Read the model definition and answer for the solid it produces. Units are mm, in the model's axes. Give positions to 0.01 mm unless a question says otherwise; leave off trailing zeros. Loops run counter-clockwise (first coordinate to the right, second up) from the corner with the lowest first, then second, coordinate; pieces in that order, holes last.
(1) Find section B-B, the plane x = 0. Write down the section's boundary in (y, z) (3 decimals).
(2) Each of these flat-tipped pins is pushed along its axis until it touches: P1, Ø5, axis at y = 3, z = 165.5, coming from the +X side; P2, Ø6, axis at y = 4, z = 248.5, coming from the +X side (3 decimals). Where does it stop, or does it pass through?
(3) Find section A-A, the plane z = 233. Write down the section's boundary in (x, y) (3 decimals).
(4) Straight lines are drawn through the part: probe 1 along Y at (x, z) = (0, 249) (3 decimals); probe 2 along Y at (x, z) = (-1, 422); probe 3 along X at (y, z) = (-2.25, 384.5). For each, find the intervals that lie inside material, in ascending order.
```python
from build123d import *

# Parameters (mm, degrees)
BOSS_EXTRUDE1_DEPTH     = 514.48335
SKETCH2_R               = 3.175
CUT_EXTRUDE1_DEPTH      = 1
CUT_EXTRUDE1_DEPTH_BACK = 515.48335


with BuildPart() as part:
    # Sketch1 → Boss-Extrude1 (new body)
    with BuildSketch(Plane.XY):
        Polygon((-7.332348419, 0), (-3.666174209, -6.35), (3.666174209, -6.35), (7.332348419, 0), (3.666174209, 6.35), (-3.666174209, 6.35), align=None)
    extrude(amount=BOSS_EXTRUDE1_DEPTH)

    # Sketch2 → Cut-Extrude1 (cut, two sides)
    with BuildSketch(Plane.XY.offset(514.48335)) as cut_extrude1_sk:
        Circle(SKETCH2_R)
    extrude(amount=CUT_EXTRUDE1_DEPTH, mode=Mode.SUBTRACT)
    extrude(cut_extrude1_sk.sketch, amount=-CUT_EXTRUDE1_DEPTH_BACK, mode=Mode.SUBTRACT)


solid = part.part
```
Entries:
1. outline: (-6.35, 0) - (-3.175, 0) - (-3.175, 514.483) - (-6.35, 514.483) - close; (3.175, 0) - (6.35, 0) - (6.35, 514.483) - (3.175, 514.483) - close
2. P1: stops at x = 7.04
2. P2: stops at x = 6.755
3. outline: (-7.332, 0) - (-3.666, -6.35) - (3.666, -6.35) - (7.332, 0) - (3.666, 6.35) - (-3.666, 6.35) - close; hole circle Ø6.35 at (0, 0)
4. probe 1: y = -6.35 to -3.175, 3.175 to 6.35
4. probe 2: y = -6.35 to -3.01, 3.01 to 6.35
4. probe 3: x = -6.03 to -2.24, 2.24 to 6.03
